from build123d import *

# Parameters (mm, degrees)
F1_W        = 864.7019863129
F1_H        = 857.8115701675
F1_R        = 74.6623748118
F2_DEPTH    = 141.6553631425
F3_T1_DEPTH = 2521.5281199611


# Not quite as in the source:
# - a fillet or chamfer that OpenCascade refuses, or shapes differently, is made with other operations: its cross-section is extruded or revolved along the edge and cut away or added


with BuildPart() as f2:
    # F1 (on face) → F2 (new body, symmetric)
    with BuildSketch(Plane.XZ):
        Rectangle(F1_W, F1_H)
        Circle(F1_R, mode=Mode.SUBTRACT)
    extrude(amount=F2_DEPTH, both=True)

    # F3: fillet of radius 447.6434787352 on 4 edges, made by hand

    # F3_s2 → F3_t1 (cut)
    with BuildSketch(Plane.XZ.offset(-1260.7640599805)):
        with BuildLine():
            ThreePointArc((-15.2924855788, 428.9057850838), (301.2392537888, 297.7940457162), (432.3509931564, -18.7376936514))
            Line((432.3509931564, -18.7376936514), (432.3509931564, 428.9057850838))
            Line((432.3509931564, 428.9057850838), (-15.2924855788, 428.9057850838))
        make_face()
        with BuildLine():
            ThreePointArc((-15.2924855788, -428.9057850838), (301.2392537888, -297.7940457162), (432.3509931564, 18.7376936514))
            Line((432.3509931564, 18.7376936514), (432.3509931564, -428.9057850838))
            Line((432.3509931564, -428.9057850838), (-15.2924855788, -428.9057850838))
        make_face()
        with BuildLine():
            ThreePointArc((15.2924855788, -428.9057850838), (-301.2392537888, -297.7940457162), (-432.3509931564, 18.7376936514))
            Line((-432.3509931564, 18.7376936514), (-432.3509931564, -428.9057850838))
            Line((-432.3509931564, -428.9057850838), (15.2924855788, -428.9057850838))
        make_face()
        with BuildLine():
            ThreePointArc((-432.3509931564, -18.7376936514), (-301.2392537888, 297.7940457162), (15.2924855788, 428.9057850838))
            Line((15.2924855788, 428.9057850838), (-432.3509931564, 428.9057850838))
            Line((-432.3509931564, 428.9057850838), (-432.3509931564, -18.7376936514))
        make_face()
    extrude(amount=F3_T1_DEPTH, mode=Mode.SUBTRACT)


solid = f2.part
Can you work these out from the model? Positions are in its coordinate system, mm. Give positions to 0.01 mm unless a question says otherwise; leave off trailing zeros. Order: outer loops, then holes, each group sorted by start corner. A loop starts at its lowest first (then second) coordinate and runs counter-clockwise, first axis right, second up. Notation, with made-up numbers: M -34,-39.5 L 22,-39.5 A18 ccw 22,-6.5 Z; hole C -6.5,63.5 d7. An arc over 180 degrees is marked long. Use a Markdown table: item, result. Add a question column.
Item 1: If I drill on L1, parallel to Z at x = 0, y = 30.5; L2, parallel to Z at x = 11.5, y = -46.5; L3, parallel to Z at x = 78.5, y = -36, over which ranges is the centre line in solid material (lowest first)? Write a range as [from, to].
Item 2: Suppose I cut it at C-C (z = 282.5). List the corners of the cut face in (x, y) for me, then the cut area to 3 significant figures.
Item 3: Suppose I cut it at D-D (x = 338). List the corners of the cut face in (y, z) for me, then the cut area to 3 significant figures.
Item 4: We'd pull the mould along Z, two halves only. Please class faces 1 (the cylindrical face through (296.68, 1.98, -302.29)), 2 (the cylindrical face through (-303.33, 1.98, 295.69)), 3 (the cylindrical face through (71.215, 1.983, 22.427)): +Z half, -Z half, draft (parallel to the pull), parting line (faces both ways), or undercut.
Item 5: Will these pins go through, and if not, where does the flat tip stop? pin 1 (12 mm diameter, centred on y = -3, z = -229.5, fed in from -X); pin 2 (10 mm diameter, centred on y = -88.5, z = 233.5, fed in from +X); pin 3 (4 mm diameter, centred on y = 64, z = -287.5, fed in from +X).
Item 6: Suppose I cut it at A-A (x = -62). List the corners of the cut face in (y, z) for me, then the cut area to 3 significant figures.
Item 7: Suppose I cut it at B-B (y = -66). List the corners of the cut face in (x, z) for me.
Answer sheet:
| question | item | result |
|---|---|---|
| 1 | L1 | z = [-428.64, -74.66], [74.66, 428.64] |
| 1 | L2 | z = [-428.1, -73.77], [73.77, 428.1] |
| 1 | L3 | z = [-418.97, 418.97] |
| 2 | outline | M -315.83,-141.66 L 315.83,-141.66 L 315.83,141.66 L -315.83,141.66 Z |
| 2 | area | 179,000 mm² |
| 3 | outline | M -141.66,-256.16 L 141.66,-256.16 L 141.66,256.16 L -141.66,256.16 Z |
| 3 | area | 145,000 mm² |
| 4 | face 1 | -Z half |
| 4 | face 2 | +Z half |
| 4 | face 3 | undercut |
| 5 | pin 1 | stops at x = -361.15 |
| 5 | pin 2 | stops at x = 357.88 |
| 5 | pin 3 | stops at x = 313.07 |
| 6 | outline | M -141.66,-422.18 L 141.66,-422.18 L 141.66,-41.6 L -141.66,-41.6 Z; M -141.66,41.6 L 141.66,41.6 L 141.66,422.18 L -141.66,422.18 Z |
| 6 | area | 216,000 mm² |
| 7 | outline | M -431.96,0 A447.64 ccw 0,-428.64 A447.64 ccw 431.96,0 A447.64 ccw 0,428.64 A447.64 ccw Z; hole C 0,0 d149.32 |
